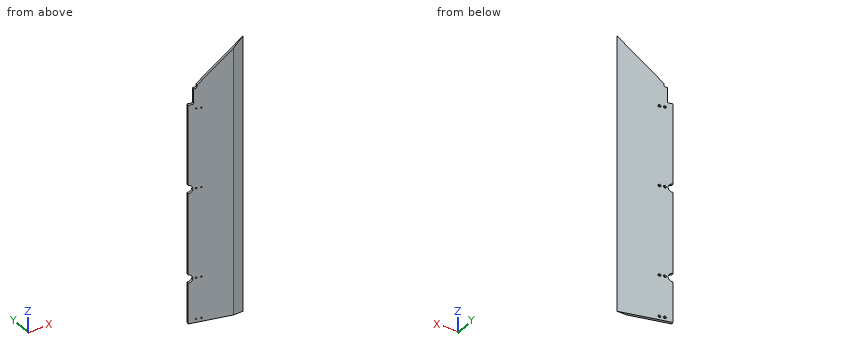
```python
from build123d import *

# Parameters (mm, degrees)
BOSS_EXTRUDE1_DEPTH                                 = 1479.55
CSK_FOR_1_4_FLAT_HEAD_SOCKET_CAP_SCREW1_D           = 7.14248
CSK_FOR_1_4_FLAT_HEAD_SOCKET_CAP_SCREW1_CSINK_D     = 13.4874
CSK_FOR_1_4_FLAT_HEAD_SOCKET_CAP_SCREW1_CSINK_ANGLE = 82
SKETCH4_R                                           = 22.225
CUT_EXTRUDE1_DEPTH                                  = 67.312434508
CUT_EXTRUDE2_DEPTH                                  = 67.312434508
FILLET1_R                                           = 6.35


with BuildPart() as part:
    # Sketch1 → Boss-Extrude1 (new body)
    with BuildSketch(Plane.XY):
        Polygon((22.225, 55.50367642), (229.367540407, 0), (278.436572382, 0), (25.512001873, 67.770934414), align=None)
    extrude(amount=BOSS_EXTRUDE1_DEPTH)

    # CSK for 1/4 Flat Head Socket Cap Screw1 (through all)
    with Locations(Plane(origin=(18.651713678, 69.609143096, 0), x_dir=(0.965925826, -0.258819045, 0), z_dir=(0.258819045, 0.965925826, 0))):
        with Locations((44.668892959, -721.51875), (70.068892959, -721.51875), (44.668892959, -240.50625), (70.068892959, -240.50625), (44.668892959, -1149.35), (70.068892959, -1149.35), (44.668892959, -19.05), (70.068892959, -19.05)):
            CounterSinkHole(CSK_FOR_1_4_FLAT_HEAD_SOCKET_CAP_SCREW1_D / 2, CSK_FOR_1_4_FLAT_HEAD_SOCKET_CAP_SCREW1_CSINK_D / 2, counter_sink_angle=CSK_FOR_1_4_FLAT_HEAD_SOCKET_CAP_SCREW1_CSINK_ANGLE)

    # Sketch4 → Cut-Extrude1 (cut, through all)
    with BuildSketch(Plane(origin=(18.651713678, 69.609143096, 0), x_dir=(0.965925826, -0.258819045, 0), z_dir=(0.258819045, 0.965925826, 0))):
        with Locations((7.102292959, -240.50625)):
            Circle(SKETCH4_R)
        with Locations((7.102292959, -721.51875)):
            Circle(SKETCH4_R)
    extrude(amount=-CUT_EXTRUDE1_DEPTH, mode=Mode.SUBTRACT)

    # Sketch5 → Cut-Extrude2 (cut, through all)
    with BuildSketch(Plane(origin=(18.651713678, 69.609143096, 0), x_dir=(0.965925826, -0.258819045, 0), z_dir=(0.258819045, 0.965925826, 0))):
        Polygon((268.949076248, -1479.55), (48.377292959, -1273.863484507), (48.377292959, -1257.3), (32.502292959, -1257.3), (32.502292959, -1174.75), (7.102292959, -1174.75), (7.102292959, -1479.55), align=None)
    extrude(amount=-CUT_EXTRUDE2_DEPTH, mode=Mode.SUBTRACT)

    # Fillet1
    fillet1_edges = [part.edges().sort_by_distance(p)[0] for p in [
        (63.737089416, 50.954549331, 1257.3),
        (48.403016924, 55.063301672, 1174.75),
    ]]
    fillet(fillet1_edges, radius=FILLET1_R)


solid = part.part
```
CAD build for the part. Positions are in the model's coordinates, mm. Round coordinates to 2 decimals unless told otherwise and drop trailing zeros. Order: outer loops, then holes, each group sorted by start corner. A loop starts at its lowest first (then second) coordinate and runs counter-clockwise, first axis right, second up.
Q1. Slice it at A-A (z = 1204.5). Write the cut outline in (x, y).
Q2. Wall check: L1, parallel to Y at x = 107, z = 236; L2, parallel to Y at x = 146, z = 1067.5; L3, parallel to Z at x = 144, y = 34. Give the ranges that are in metal, low to high.
Q3. Slice it at B-B (x = 155). Write the cut outline in (y, z), and give its area (3 significant figures).
Q4. Drop flat-ended pins along their axis: pin 1 (3 mm diameter, centred on x = 131, z = 239, fed in from +Y); pin 2 (8 mm diameter, centred on x = 68, z = 234, fed in from -Y); pin 3 (5 mm diameter, centred on y = 55, z = 1039.5, fed in from -X) (3 decimals). Give the stop position or say it passes through.
Results below:
1. outline: (46.76, 48.93) - (229.37, 0) - (278.44, 0) - (50.05, 61.2) - close
2. L1: y = 32.79 to 45.94
2. L2: y = 22.34 to 35.49
2. L3: z = 0 to 1350.25
3. outline: (19.93, 0) - (33.07, 0) - (33.07, 1360.38) - (19.93, 1363.56) - close
3. area: 17,900 mm2
4. pin 1: stops at y = 39.91
4. pin 2: stops at y = 42.17
4. pin 3: stops at x = 22.225
